Source: CAD feature listing. Evaluate the final solid. Frame: model axes, mm. A direction names the side the tool comes from. Round coordinates to 2 decimals unless told otherwise and drop trailing zeros. Order: outer loops, then holes, each group sorted by start corner. A loop starts at its lowest first (then second) coordinate and runs counter-clockwise, first axis right, second up. Notation, with made-up numbers: M 25.25,-32 L 78.25,-32 A11 cw 78.25,-18 Z; hole C 89.25,-21 d3. An arc over 180 degrees is marked long. Use one line per item in the form item = value. Start each with the question number.
Q1. Reachability of faces 4 (the flat face through (-1, -1, 0)), 5 (the flat face through (0.51, -0.86, -1.76)), 6 (the flat face through (-1, -1, -2.5)) from +Z, -Z, +X, -X, +Y, -Y: full face, straight path, thin tool, end or side. Return the list, or none.
Q2. Section A-A (y = 0). Return the cut outline in (x, z).
Q3. Material intervals for probe 1 along Z at (x, y) = (1.2, 0.9); probe 2 along Z at (x, y) = (-0.8, 0.35); probe 3 along Y at (x, z) = (0.4, -1.25), sorted ascending.
Q4. Contact query for flat-ended pins moving along their axis: pin 1 (1.3 mm diameter, centred on y = 0.5, z = -2, fed in from +X); pin 2 (2 mm diameter, centred on y = 1.5, z = 5, fed in from +X). Output: stop coordinate, or through.
Q5. Pull-direction query (Y, two-part tool) for faces 1 (the flat face through (0, 0, 16)), 2 (the flat face through (0, 0, -1)), 3 (the cylindrical face through (0.29, 2.23, -1.06)); classes: pulls with the +Y half, pulls with the -Y half, needs draft (parallel to the pull), parting line crosses it, or undercut.
Q6. Section B-B (z = -0.25). Return the cut outline in (x, y).
from build123d import *

# Parameters (mm, degrees)
CROQUIS1_R              = 1.25
SALIENTE_EXTRUIR1_DEPTH = 16
CROQUIS2_R              = 2.25
SALIENTE_EXTRUIR2_DEPTH = 2.5
CORTAR_EXTRUIR1_DEPTH   = 1.5
REDONDEO1_R             = 0.35


with BuildPart() as part:
    # Croquis1 → Saliente-Extruir1 (new body)
    with BuildSketch(Plane.XY):
        Circle(CROQUIS1_R)
    extrude(amount=SALIENTE_EXTRUIR1_DEPTH)

    # Croquis2 → Saliente-Extruir2 (add)
    with BuildSketch(Plane(origin=(0, 0, 0), x_dir=(-1, 0, 0), z_dir=(0, 0, -1))):
        Circle(CROQUIS2_R)
    extrude(amount=SALIENTE_EXTRUIR2_DEPTH)

    # Croquis3 → Cortar-Extruir1 (cut)
    with BuildSketch(Plane(origin=(0, 0, -2.5), x_dir=(-1, 0, 0), z_dir=(0, 0, -1))):
        Polygon((0, -1.154700538), (1, -0.577350269), (1, 0.577350269), (0, 1.154700538), (-1, 0.577350269), (-1, -0.577350269), align=None)
    extrude(amount=-CORTAR_EXTRUIR1_DEPTH, mode=Mode.SUBTRACT)

    # Redondeo1
    redondeo1_edges = [part.edges().sort_by_distance(p)[0] for p in [
        (2.25, 0, -2.5),
    ]]
    fillet(redondeo1_edges, radius=REDONDEO1_R)


solid = part.part
Results list:
q1.face_4 = +Z
q1.face_5 = -Z
q1.face_6 = -Z, +X, -X, +Y, -Y
q2.outline = M -2.25,-2.15 A0.35 ccw -1.9,-2.5 L -1,-2.5 L -1,-1 L 1,-1 L 1,-2.5 L 1.9,-2.5 A0.35 ccw 2.25,-2.15 L 2.25,0 L 1.25,0 L 1.25,16 L -1.25,16 L -1.25,0 L -2.25,0 Z
q3.probe_1 = -2.5 to 0
q3.probe_2 = -1 to 16
q3.probe_3 = -2.21 to -0.92, 0.92 to 2.21
q4.pin_1 = 2.25
q4.pin_2 = 1.15
q5.face_1 = needs draft
q5.face_2 = undercut
q5.face_3 = parting line crosses it
q6.outline = C 0,0 d4.5
